Part print with two shaded views. Sizes in mm from the minimum x, y, z corner. Give positions to 0.01 mm unless a question says otherwise; leave off trailing zeros. Write each loop counter-clockwise with the first axis right and the second up, starting at its lowest first coordinate (ties: lowest second). Pieces come first, ordered by that corner, then holes.
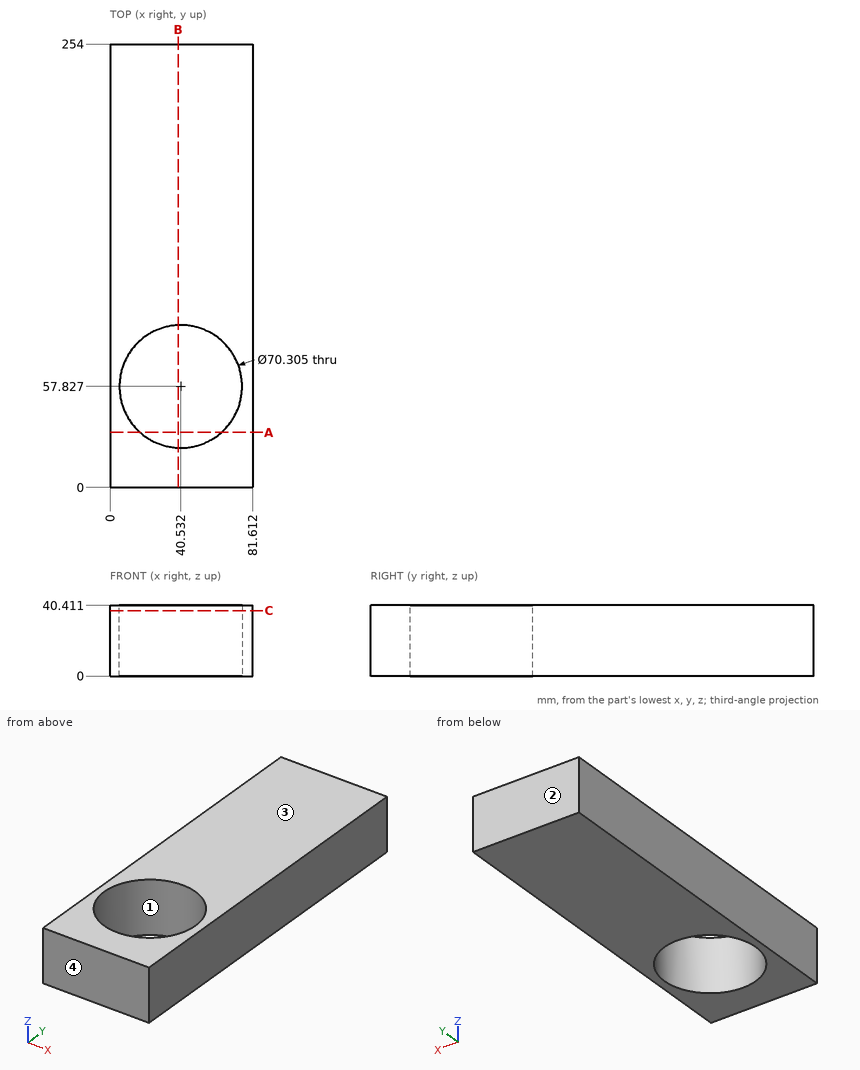
1) Drill centre lines: L1, parallel to X at y = 71.5, z = 19.5; L2, parallel to X at y = 48.5, z = 4.5 (1 decimal); L3, parallel to Y at x = 11, z = 19.5 (1 decimal). Where is each one in solid material? Low to high.
Check result:
L1: x = 0 to 8.15, 72.92 to 81.61
L2: x = 0 to 6.6, 74.4 to 81.6
L3: y = 0 to 38.8, 76.9 to 254
2) Saw through at A-A (y = 31.5). Write the cut outline in (x, z) (1 decimal), and give its area (3 significant figures).
Check result:
outline: (0, 0) - (17.2, 0) - (17.2, 40.4) - (0, 40.4) - close; (63.8, 0) - (81.6, 0) - (81.6, 40.4) - (63.8, 40.4) - close
area: 1,420 mm2
3) Saw through at B-B (x = 39). Write the cut outline in (y, z).
Check result:
outline: (0, 0) - (22.71, 0) - (22.71, 40.41) - (0, 40.41) - close; (92.95, 0) - (254, 0) - (254, 40.41) - (92.95, 40.41) - close
4) Mould opens along Y. For the marked faces 1, 2, 3 and 4 say: +Y half, -Y half, draft (parallel to the pull), parting line (faces both ways), or undercut.
Check result:
face 1: undercut
face 2: +Y half
face 3: draft
face 4: -Y half
5) Flat gauge pin, fed straight in: P1, Ø1, axis at x = 27.5, z = 10, coming from the -Y side. Where does the tip first touch, or does it go through?
Check result:
P1: stops at y = 0
6) Saw through at C-C (z = 37.5). Write the cut outline in (x, y) (1 decimal), and give its area (3 significant figures).
Check result:
outline: (0, 0) - (81.6, 0) - (81.6, 254) - (0, 254) - close; hole circle Ø70.3 at (40.5, 57.8)
area: 16,800 mm2
